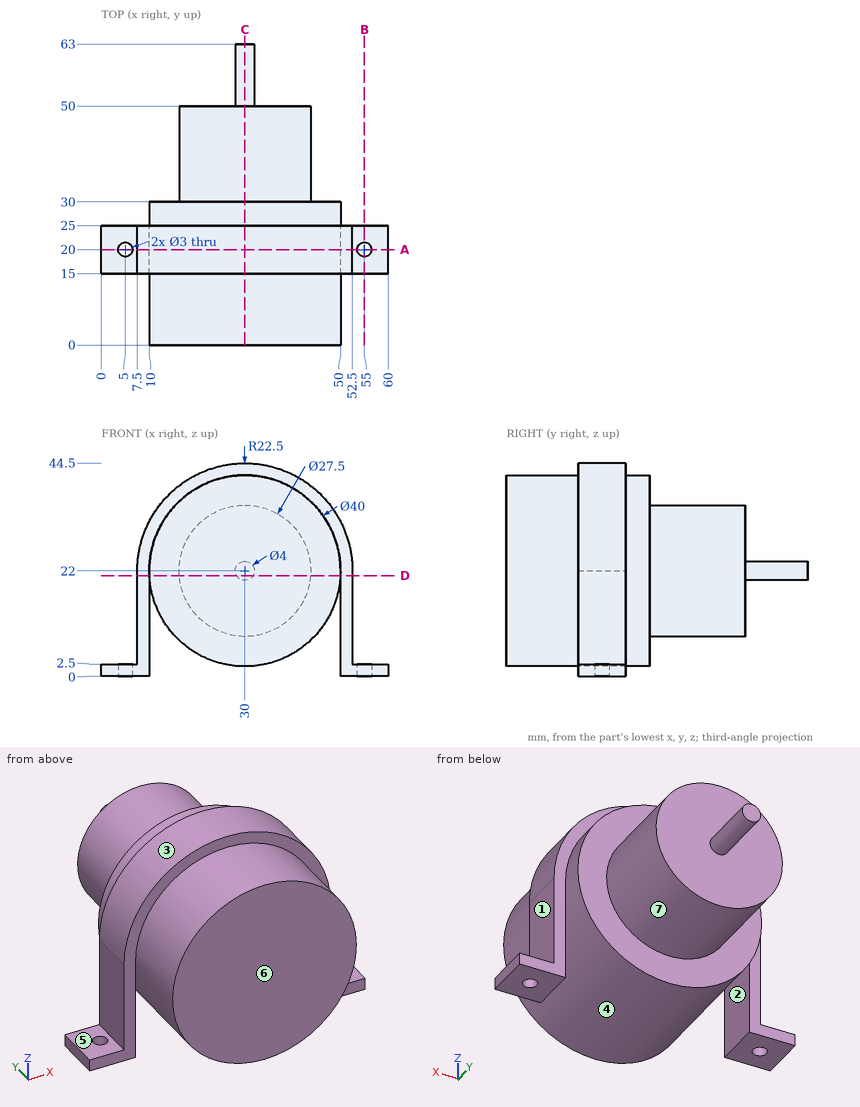
Study the drawing (mm; zero at the part's minimum x, y, z) and answer. A direction names the side the tool comes from. Give positions to 0.01 mm unless a question says otherwise; leave off trailing zeros. Write each loop counter-clockwise with the first axis right and the second up, starting at its lowest first coordinate (ties: lowest second). Pieces come first, ordered by that corner, then holes.
(1) Straight lines are drawn through the part: line 1 (Y direction, x = 5, z = 1); line 2 (X direction, y = 17, z = 4); line 3 (Y direction, x = 31, z = 11.5). For each, find the intervals that lie inside material, in ascending order.
Final values:
line 1: y = 15 to 18.5, 21.5 to 25
line 2: x = 7.5 to 10, 21.28 to 38.72, 50 to 52.5
line 3: y = 0 to 50
(2) The part is cut by section B-B on x = 55. Write down the section's boundary in (y, z), plus the area to 3 significant figures.
Final values:
outline: (15, 0) - (18.5, 0) - (18.5, 2.5) - (15, 2.5) - close; (21.5, 0) - (25, 0) - (25, 2.5) - (21.5, 2.5) - close
area: 17.5 mm2
(3) The mould has two halves that part along X. Classify the marked faces 1, 2, 3 and 4: pulls with the +X half, pulls with the -X half, needs draft (parallel to the pull), parting line crosses it, or undercut.
Final values:
face 1: pulls with the +X half
face 2: undercut
face 3: parting line crosses it
face 4: undercut
(4) Flat-ended cylindrical pins translate along their axes: pin 1 Ø4 at (y, z) = (17.5, 20.5) entering from +X; pin 2 Ø12 at (y, z) = (23.5, 23) entering from -X; pin 3 Ø1.5 at (x, z) = (11, 9.5) entering from +Y; pin 4 Ø4 at (x, y) = (3.5, 21.5) entering from +Z. Find the tip coordinate at first contact, or state that the pin passes through.
Final values:
pin 1: stops at x = 52.5
pin 2: stops at x = 7.5
pin 3: passes through
pin 4: stops at z = 2.5
(5) The part is cut by section C-C on x = 30. Write down the section's boundary in (y, z), plus the area to 3 significant figures.
Final values:
outline: (0, 2) - (30, 2) - (30, 8.25) - (50, 8.25) - (50, 20) - (63, 20) - (63, 24) - (50, 24) - (50, 35.75) - (30, 35.75) - (30, 42) - (25, 42) - (25, 44.5) - (15, 44.5) - (15, 42) - (0, 42) - close
area: 1,830 mm2
(6) The part is cut by section A-A on y = 20. Write down the section's boundary in (x, z), plus the area to 3 significant figures.
Final values:
outline: (0, 0) - (3.5, 0) - (3.5, 2.5) - (0, 2.5) - close; (6.5, 0) - (10, 0) - (10, 22) arc R20 ccw to (50, 22) - (50, 0) - (53.5, 0) - (53.5, 2.5) - (52.5, 2.5) - (52.5, 22) arc R22.5 ccw to (7.5, 22) - (7.5, 2.5) - (6.5, 2.5) - close; (56.5, 0) - (60, 0) - (60, 2.5) - (56.5, 2.5) - close
area: 1,560 mm2
(7) The part is cut by section D-D on z = 21. Write down the section's boundary in (x, y).
Final values:
outline: (7.5, 15) - (10, 15) - (10, 25) - (7.5, 25) - close; (10.03, 0) - (49.97, 0) - (49.97, 30) - (43.71, 30) - (43.71, 50) - (31.73, 50) - (31.73, 63) - (28.27, 63) - (28.27, 50) - (16.29, 50) - (16.29, 30) - (10.03, 30) - close; (50, 15) - (52.5, 15) - (52.5, 25) - (50, 25) - close
(8) Which of the six approach directions +Z, -Z, +X, -X, +Y, -Y give full straight-line access (tool end or side, diameter ignored) to the marked faces 5, 6 and 7?
Final values:
face 5: +Z, -X, +Y, -Y
face 6: +Z, -Z, +X, -X, -Y
face 7: +Y
